Design review of the part shown in the three views and the two pictorial views. Dimensions are in mm from the part's minimum x, y and z. A direction names the side the tool comes from. Coordinates: 2 decimals unless noted, no trailing zeros. Loops run counter-clockwise (first coordinate to the right, second up) from the corner with the lowest first, then second, coordinate; pieces in that order, holes last.
Q1. Add section C-C on y = 9. Give the boundary of the cut face in (x, z).
Q2. Wall thickness on probe 1 along Y at (x, z) = (11, 7.25); probe 2 along Y at (x, z) = (18.5, 6.5); probe 3 along X at (y, z) = (20, 7.75): over which ranges is each line inside the solid? List them lowest first.
Q3. For P1, Ø6, axis at y = 5, z = 3.5, coming from the +X side; P2, Ø1.9, axis at x = 2, z = 9.5, coming from the +Y side; P3, Ø2.5, axis at x = 24.5, z = 8, coming from the -Y side, all flat-tipped, find the tip position at first contact; note any pin that passes through.
Q4. Add section B-B on x = 20.5. Give the boundary of the cut face in (y, z), and give its area (3 significant figures).
Q5. Add section A-A on z = 11.25. Give the boundary of the cut face in (x, y).
Q6. Machinability: for the marked faces 1, 2 and 3, which of the approach directions +Z, -Z, +X, -X, +Y, -Y give a long, thin tool a straight path to every point of the face, cutting with its end or side? Answer none if there is none.
Q7. Add section D-D on z = 2.25. Give the boundary of the cut face in (x, y).
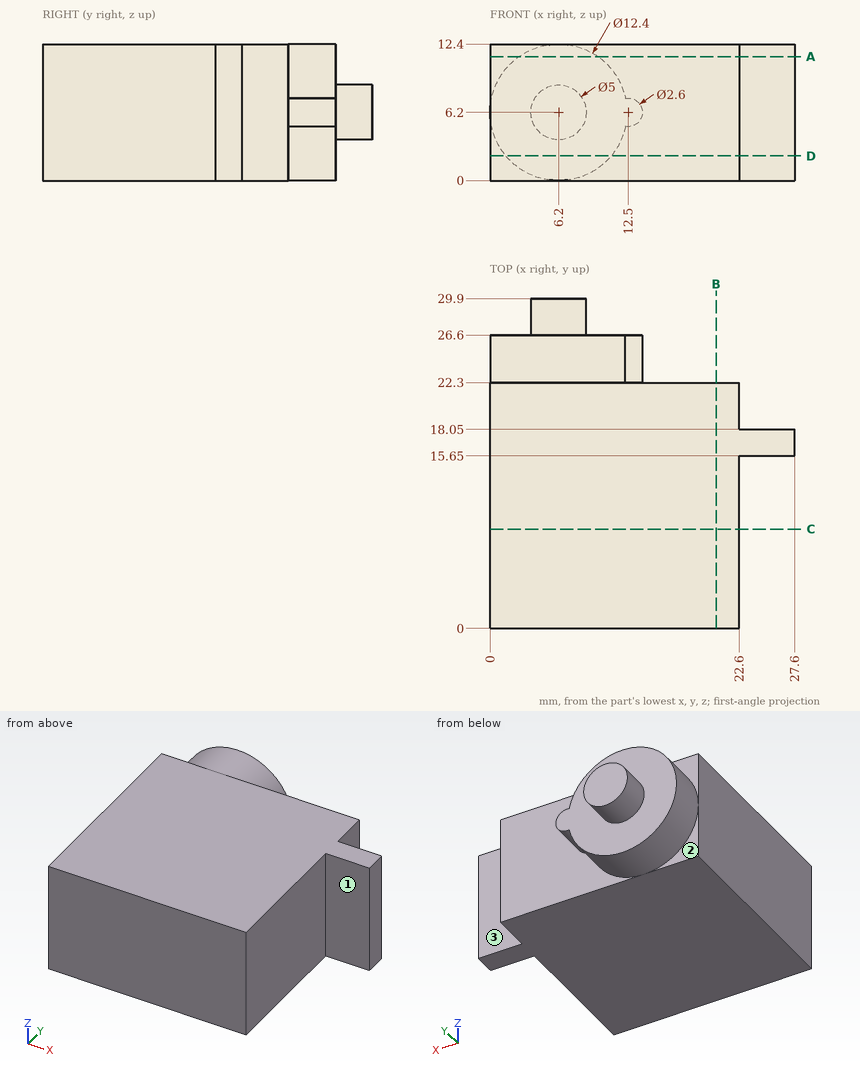
Entries:
1. outline: (0, 0) - (22.6, 0) - (22.6, 12.4) - (0, 12.4) - close
2. probe 1: y = 0 to 26.6
2. probe 2: y = 0 to 22.3
2. probe 3: x = 0 to 22.6
3. P1: stops at x = 22.6
3. P2: stops at y = 26.6
3. P3: stops at y = 15.65
4. outline: (0, 0) - (22.3, 0) - (22.3, 12.4) - (0, 12.4) - close
4. area: 277 mm2
5. outline: (0, 0) - (22.6, 0) - (22.6, 15.65) - (27.6, 15.65) - (27.6, 18.05) - (22.6, 18.05) - (22.6, 22.3) - (9.8, 22.3) - (9.8, 26.6) - (2.6, 26.6) - (2.6, 22.3) - (0, 22.3) - close
6. face 1: +Z, -Z, +X, -Y
6. face 2: -Z, -X, +Y
6. face 3: +Z, -Z, +X, +Y
7. outline: (0, 0) - (22.6, 0) - (22.6, 15.65) - (27.6, 15.65) - (27.6, 18.05) - (22.6, 18.05) - (22.6, 22.3) - (10.98, 22.3) - (10.98, 26.6) - (1.42, 26.6) - (1.42, 22.3) - (0, 22.3) - close
